Study the drawing (mm; zero at the part's minimum x, y, z) and answer. Coordinates: 2 decimals unless noted, no trailing zeros. Loops run counter-clockwise (first coordinate to the right, second up) from the corner with the lowest first, then second, coordinate; pieces in that order, holes last. Notation, with made-up numbers: M -2,18.5 L 10,18.5 A16 cw 10,31.5 Z; hole C 42,79.25 d7. An arc over 180 degrees is marked long. Use one line per item in the form item = value. Start each with the question number.
1. For a pull along Y with two mould halves and no side action, classify the marked faces 1, 2 and 3 as released by +Y, released by -Y, zero draft, split by the parting line, or undercut.
2. The part is cut by section A-A (z = 38). Give the vertices of the cut face in (x, y).
3. Find the intervals of material crossed by probe 1 along Y at (x, z) = (85, 34); probe 2 along Y at (x, z) = (9, 37.5); probe 3 along X at (y, z) = (0.75, 30), in increasing order. Write a range as [from, to].
4. The part is cut by section C-C (x = 29). Give the vertices of the cut face in (y, z), plus the area to 4 significant figures.
5. The part is cut by section B-B (y = 9). Give the vertices of the cut face in (x, z).
6. Flat-ended cylindrical pins translate along their axes: pin 1 (0.8 mm diameter, centred on x = 4.5, y = 1, fed in from -Z); pin 2 (5 mm diameter, centred on y = 7.5, z = 42.5, fed in from +X); pin 3 (2 mm diameter, centred on x = 140, y = 2, fed in from +Z). Find the tip coordinate at first contact, or state that the pin passes through.
7. The part is cut by section D-D (z = 70). Give the vertices of the cut face in (x, y).
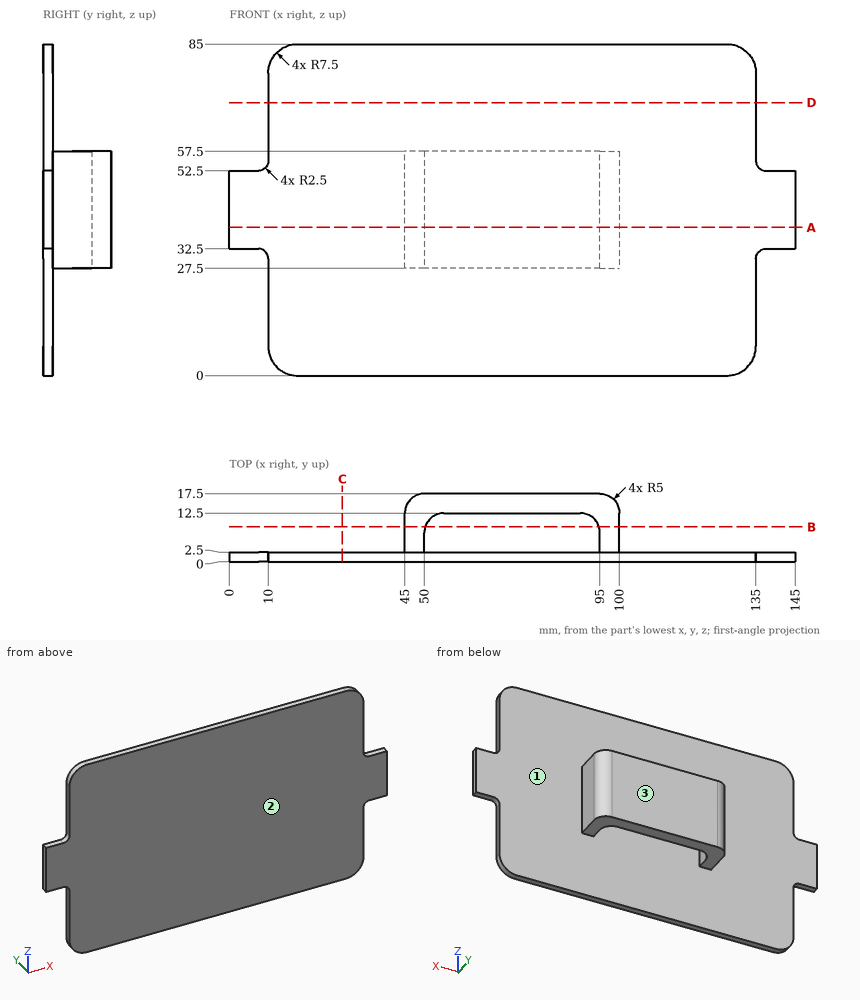
Computed values:
q1.face_1 = undercut
q1.face_2 = released by -Y
q1.face_3 = released by +Y
q2.outline = M 0,0 L 145,0 L 145,2.5 L 100,2.5 L 100,12.5 A5 ccw 95,17.5 L 50,17.5 A5 ccw 45,12.5 L 45,2.5 L 0,2.5 Z; hole M 50,2.5 L 95,2.5 L 95,7.5 A5 ccw 90,12.5 L 55,12.5 A5 ccw 50,7.5 Z
q3.probe_1 = [0, 2.5], [12.5, 17.5]
q3.probe_2 = [0, 2.5]
q3.probe_3 = [10, 135]
q4.outline = M 0,0 L 2.5,0 L 2.5,85 L 0,85 Z
q4.area = 212.5 mm²
q5.outline = M 45,27.5 L 50.23,27.5 L 50.23,57.5 L 45,57.5 Z; M 94.77,27.5 L 100,27.5 L 100,57.5 L 94.77,57.5 Z
q6.pin_1 = 32.5
q6.pin_2 = 100
q6.pin_3 = 52.5
q7.outline = M 10,0 L 135,0 L 135,2.5 L 10,2.5 Z
